```python
from build123d import *

# Parameters (mm, degrees)
CROQUIS1_W              = 254
CROQUIS1_H              = 152.4
CROQUIS1_R              = 2
CROQUIS1_R_2            = 7
SALIENTE_EXTRUIR1_DEPTH = 10
CROQUIS2_R              = 2
CORTAR_EXTRUIR1_DEPTH   = 10
CROQUIS3_W              = 254
CROQUIS3_H              = 20
SALIENTE_EXTRUIR2_DEPTH = 20


with BuildPart() as part:
    # Croquis1 → Saliente-Extruir1 (new body)
    with BuildSketch(Plane.XY):
        with Locations((1.935502346, -46)):
            Rectangle(CROQUIS1_W, CROQUIS1_H)
        with Locations((38.725502346, -81)):
            Circle(CROQUIS1_R, mode=Mode.SUBTRACT)
        with Locations((-43.314497654, -46)):
            Circle(CROQUIS1_R_2, mode=Mode.SUBTRACT)
        with BuildLine():
            Line((-19.767986026, -36.106195294), (64.415153509, -23.738939412))
            ThreePointArc((64.415153509, -23.738939412), (82.393784897, -28.973067674), (90.185502346, -46))
            ThreePointArc((90.185502346, -46), (82.393784897, -63.026932326), (64.415153509, -68.261060588))
            Line((64.415153509, -68.261060588), (-19.767986026, -55.893804706))
            ThreePointArc((-19.767986026, -55.893804706), (-28.314497654, -46), (-19.767986026, -36.106195294))
        make_face(mode=Mode.SUBTRACT)
        with Locations((38.725502346, -11)):
            Circle(CROQUIS1_R, mode=Mode.SUBTRACT)
    extrude(amount=SALIENTE_EXTRUIR1_DEPTH)

    # Croquis2 → Cortar-Extruir1 (cut)
    with BuildSketch(Plane.XY.offset(10)):
        with Locations((-115.064497654, 20.2)):
            Circle(CROQUIS2_R)
        with Locations(Location((118.935502346, 20.2, 0), (0, 0, 180))):
            Circle(CROQUIS2_R)
    extrude(amount=-CORTAR_EXTRUIR1_DEPTH, mode=Mode.SUBTRACT)

    # Croquis3 → Saliente-Extruir2 (add)
    with BuildSketch(Plane.XY.offset(10)):
        with Locations((1.935502346, -75)):
            Rectangle(CROQUIS3_W, CROQUIS3_H)
    extrude(amount=SALIENTE_EXTRUIR2_DEPTH)


solid = part.part
```
Geometry: final body of the model. Coordinates: model frame, mm. A direction names the side the tool comes from. Coordinates: 2 decimals unless noted, no trailing zeros. Write each loop counter-clockwise with the first axis right and the second up, starting at its lowest first coordinate (ties: lowest second). Pieces come first, ordered by that corner, then holes. Notation, with made-up numbers: M -3.75,-36 L 43.25,-36 A26 cw 43.25,0 Z; hole C 79.5,76.5 d5. An arc over 180 degrees is marked long. Answer as CSV lines item,"result". Start each with the question number.
Q1. Line query: line 1 (X direction, y = -49, z = 7.25); line 2 (Z direction, x = -90.5, y = -41); line 3 (Y direction, x = 70, z = 6.5). Output: solid intervals per line, ascending. Write a range as from..to.
Q2. Pin query (flat end, axial travel): P1, Ø1.1, axis at x = 63.5, y = -66, coming from the -Z side; P2, Ø18, axis at x = -43.31, y = -46, coming from the +Z side; P3, Ø10, axis at x = 84.5, z = 12, coming from the +Y side; P4, Ø6, axis at x = -60.5, z = 24.5, coming from the -Y side. Return the tip coordinate at first contact, or that it passes through.
Q3. Mould query, pull axis X, two halves, no side actions, for faces 6 (the flat face through (22.913, -62.164, 4.93)), 7 (the flat face through (-125.064, -47, 8)), 8 (the flat face through (0, -85, 20)). Classes: released by +X, released by -X, zero draft, split by the parting line, or undercut.
Q4. Cut plane A-A on x = -14.5. Return the cut outline in (y, z), then the cut area to 3 significant figures.
Q5. Cut plane D-D on z = 25. Return the cut outline in (x, y), then the cut area to 3 significant figures.
Q6. Reachability of faces 1 (the flat face through (0, -103, 10)), 2 (the flat face through (0, -28, 0)), 3 (the flat face through (0, -65, 20)), 4 (the flat face through (0, 30.2, 5)), 5 (the flat face through (21.73, -30.01, 4.93)) from +Z, -Z, +X, -X, +Y, -Y: full face, straight path, thin tool, end or side. Return the list, or none.
Q7. Cut plane C-C on x = -76. Return the cut outline in (y, z), then the cut area to 3 significant figures.
Q8. Cut plane B-B on y = -43.5. Return the cut outline in (x, z).
Findings below:
1,line 1,"x = -125.06..-49.64, -36.99..-27.85, 89.98..128.94"
1,line 2,"z = 0..10"
1,line 3,"y = -122.2..-68.38, -23.62..30.2"
2,P1,"stops at z = 10"
2,P2,"stops at z = 10"
2,P3,"stops at y = 30.2"
2,P4,"stops at y = -85"
3,face 6,"undercut"
3,face 7,"released by -X"
3,face 8,"zero draft"
4,outline,"M -122.2,0 L -56.67,0 L -56.67,10 L -65,10 L -65,30 L -85,30 L -85,10 L -122.2,10 Z; M -35.33,0 L 30.2,0 L 30.2,10 L -35.33,10 Z"
4,area,"1,710 mm2"
5,outline,"M -125.06,-85 L 128.94,-85 L 128.94,-65 L -125.06,-65 Z"
5,area,"5,080 mm2"
6,face 1,"+Z, +X, -X, -Y"
6,face 2,"-Z, +X, -X, +Y, -Y"
6,face 3,"+Z, +X, -X, +Y"
6,face 4,"+Z, -Z, +X, -X, +Y"
6,face 5,"+Z, -Z"
7,outline,"M -122.2,0 L 30.2,0 L 30.2,10 L -65,10 L -65,30 L -85,30 L -85,10 L -122.2,10 Z"
7,area,"1,920 mm2"
8,outline,"M -125.06,0 L -49.85,0 L -49.85,10 L -125.06,10 Z; M -36.78,0 L -28,0 L -28,10 L -36.78,10 Z; M 90.05,0 L 128.94,0 L 128.94,10 L 90.05,10 Z"
